```python
from build123d import *

# Parameters (mm, degrees)
F0_W     = 22.55
F0_H     = 22.55
F0_W_2   = 16.55
F0_H_2   = 16.55
F1_DEPTH = 5
F2_DEPTH = 15
F3_SIZE  = 2


with BuildPart() as f1:
    # F0 (on Top) → F1 (new body)
    with BuildSketch(Plane.XY):
        with Locations((-8.275, 8.275)):
            Rectangle(F0_W, F0_H)
        with Locations((-8.275, 8.275)):
            Rectangle(F0_W_2, F0_H_2, mode=Mode.SUBTRACT)
    extrude(amount=F1_DEPTH)

    # F0 (on Top) → F2 (join)
    with BuildSketch(Plane.XY):
        with Locations((-8.275, 8.275)):
            Rectangle(F0_W, F0_H)
        with Locations((-8.275, 8.275)):
            Rectangle(F0_W_2, F0_H_2, mode=Mode.SUBTRACT)
    extrude(amount=F2_DEPTH)

    # F3
    f3_edges = [f1.edges().sort_by_distance(p)[0] for p in [
        (-8.275, 16.55, 15),
        (-16.55, 8.275, 15),
        (0, 8.275, 15),
        (-8.275, 0, 15),
    ]]
    chamfer(f3_edges, length=F3_SIZE)


solid = f1.part
```
Input: part model. Units: mm. Frame: model coordinates. A direction names the side the tool comes from. Coordinates: 2 decimals unless noted, no trailing zeros. Write each loop counter-clockwise with the first axis right and the second up, starting at its lowest first coordinate (ties: lowest second). Pieces come first, ordered by that corner, then holes. Notation, with made-up numbers: (71, -11) - (113, -11) arc R17 cw to (113, -6) - close; hole circle Ø1 at (-6.75, 50.5). An arc over 180 degrees is marked (long way). Put each result on its own line as item: value. Start each with the question number.
1) Cut plane A-A (z = 3.5). Return the cut outline in (x, y), plus the area to 3 significant figures.
2) Cut plane B-B (x = -8). Return the cut outline in (y, z), plus the area to 3 significant figures.
3) Cut plane D-D (x = 0.5). Return the cut outline in (y, z), plus the area to 3 significant figures.
4) Ray query, L1, parallel to X at y = 5, z = 6.5; L2, parallel to Y at x = -7.5, z = 11.5; L3, parallel to X at y = 6.5, z = 14.25. Return the intervals inside material, ascending.
5) Mould query, pull axis X, two halves, no side actions, for faces 4 (the face through (-8, -3, 7)), 5 (the face through (1, 8, 14)), 6 (the face through (-8, 0, 6)), 7 (the face through (3, 8, 7)). Classes: pulls with the +X half, pulls with the -X half, needs draft (parallel to the pull), parting line crosses it, or undercut.
6) Reachability of faces 1 (the face through (-8, -1, 14)), 2 (the face through (-16.55, 8, 6)), 3 (the face through (-18, 8, 0)) from +Z, -Z, +X, -X, +Y, -Y: full face, straight path, thin tool, end or side. Return the list, or none.
7) Cut plane C-C (y = 6). Return the cut outline in (x, z), plus the area to 3 significant figures.
Resolved:
1. outline: (-19.55, -3) - (3, -3) - (3, 19.55) - (-19.55, 19.55) - close; hole (-16.55, 0) - (0, 0) - (0, 16.55) - (-16.55, 16.55) - close
1. area: 235 mm2
2. outline: (-3, 0) - (0, 0) - (0, 13) - (-2, 15) - (-3, 15) - close; (16.55, 0) - (19.55, 0) - (19.55, 15) - (18.55, 15) - (16.55, 13) - close
2. area: 86.0 mm2
3. outline: (-3, 0) - (19.55, 0) - (19.55, 15) - (18.55, 15) - (17.05, 13.5) - (-0.5, 13.5) - (-2, 15) - (-3, 15) - close
3. area: 310 mm2
4. L1: x = -19.55 to -16.55, 0 to 3
4. L2: y = -3 to 0, 16.55 to 19.55
4. L3: x = -19.55 to -17.8, 1.25 to 3
5. face 4: needs draft
5. face 5: undercut
5. face 6: undercut
5. face 7: pulls with the +X half
6. face 1: +Z
6. face 2: +Z, -Z
6. face 3: -Z, +X, -X, +Y, -Y
7. outline: (-19.55, 0) - (-16.55, 0) - (-16.55, 13) - (-18.55, 15) - (-19.55, 15) - close; (0, 0) - (3, 0) - (3, 15) - (2, 15) - (0, 13) - close
7. area: 86.0 mm2
